Check sheet for the drawn part. Datum: minimum x, y, z corner. Units: mm. A direction names the side the tool comes from. Coordinates: 2 decimals unless noted, no trailing zeros. Write each loop counter-clockwise with the first axis right and the second up, starting at its lowest first coordinate (ties: lowest second). Pieces come first, ordered by that corner, then holes. Notation, with made-up numbers: (0.25, -21.75) -> (46.25, -21.75) arc R13 cw to (46.25, -5.75) -> close; hole circle Ø10 at (59.25, 68). An arc over 180 degrees is marked (long way). Answer in a Markdown table with one row per item. Add a question column.
1. Set-up check for the marked faces 1 and 2: record each of +Z, -Z, +X, -X, +Y, -Y from which the full face is reachable in a straight line by a thin tool's end or side.
2. Depth check by flat-ended pin: P1, Ø4.5, axis at y = 18, z = 15.5, coming from the +X side; P2, Ø3, axis at y = 26.5, z = 7, coming from the +X side; P3, Ø1.2, axis at x = 22.5, z = 12, coming from the -Y side; P4, Ø10, axis at x = 10, y = 25.5, coming from the +Z side. Enter the tip coordinate at first touch or a pass-through.
3. Cross-section at C-C on y = 31. Record the cut outline in (x, z), and give its area (3 significant figures).
4. Mould release check, pull along Y, two halves, no side actions. Record for the marked faces 3, 4 and 5: pulls with the +Y half, pulls with the -Y half, needs draft (parallel to the pull), parting line crosses it, or undercut.
5. Cross-section at B-B on y = 9.5. Record the cut outline in (x, z).
6. Cross-section at A-A on x = 12. Record the cut outline in (y, z).
7. Scan lines: L1, parallel to Z at x = 12.25, y = 9.5; L2, parallel to Y at x = 22.25, z = 10.75; L3, parallel to Z at x = 9, y = 9.5. Record each from-to range of solid material in increasing order. Write a range as from..to.
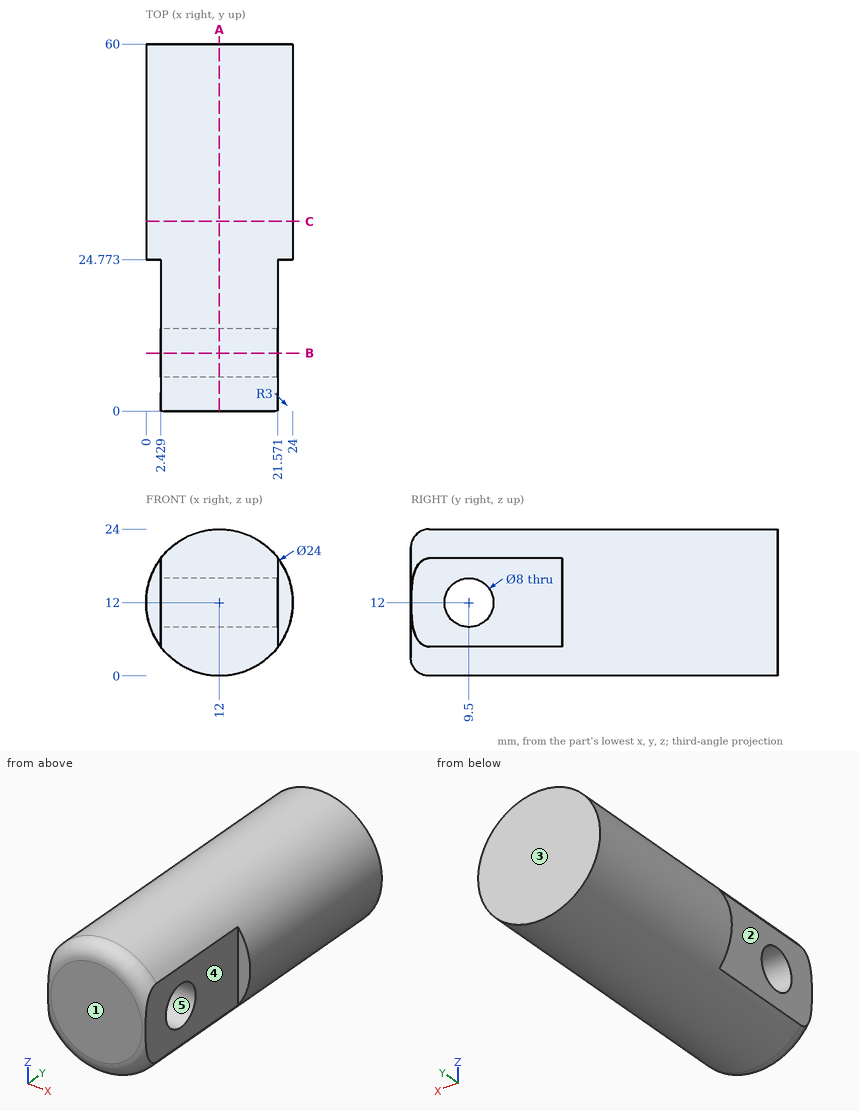
Results found:
| question | item | result |
|---|---|---|
| 1 | face 1 | +Z, -Z, +X, -X, -Y |
| 1 | face 2 | +Z, -Z, -X, -Y |
| 2 | P1 | stops at x = 21.57 |
| 2 | P2 | stops at x = 23.48 |
| 2 | P3 | stops at y = 24.77 |
| 2 | P4 | stops at z = 24 |
| 3 | outline | circle Ø24 at (12, 12) |
| 3 | area | 452 mm^2 |
| 4 | face 3 | pulls with the +Y half |
| 4 | face 4 | needs draft |
| 4 | face 5 | undercut |
| 5 | outline | (2.43, 4.76) arc R12 ccw to (21.57, 4.76) -> (21.57, 8) -> (2.43, 8) -> close; (2.43, 16) -> (21.57, 16) -> (21.57, 19.24) arc R12 ccw to (2.43, 19.24) -> close |
| 6 | outline | (0, 3) arc R3 ccw to (3, 0) -> (60, 0) -> (60, 24) -> (3, 24) arc R3 ccw to (0, 21) -> close; hole circle Ø8 at (9.5, 12) |
| 7 | L1 | z = 0..8, 16..24 |
| 7 | L2 | y = 24.77..60 |
| 7 | L3 | z = 0.38..8, 16..23.62 |
